Check sheet for the modelled part. Datum: model origin and axes. Units: mm. Face numbers are marked on the shaded views. A direction names the side the tool comes from. Give positions to 0.01 mm unless a question says otherwise; leave off trailing zeros. Order: outer loops, then holes, each group sorted by start corner. A loop starts at its lowest first (then second) coordinate and runs counter-clockwise, first axis right, second up. Notation, with made-up numbers: (19, 49) - (36, 49) arc R24 ccw to (36, 71) - close; hole circle Ø2 at (63.5, 32). An arc over 180 degrees is marked (long way). Answer in a Markdown table with one row per item.
from build123d import *

# Parameters (mm, degrees)
F1_DEPTH = 41.275
F0_W     = 25.4
F0_H     = 19.05
F2_DEPTH = 22.225
F4_DEPTH = 12.7
F5_R     = 6.35


with BuildPart() as f1:
    # F0 (on Front) → F1 (new body, symmetric)
    with BuildSketch(Plane.XZ):
        Polygon((-41.275, 9.525), (-41.275, -9.525), (41.275, -9.525), (41.275, 9.525), (22.225, 9.525), align=None)
    extrude(amount=F1_DEPTH, both=True)

    # F0 (on Front) → F2 (join, symmetric)
    with BuildSketch(Plane.XZ):
        with BuildLine():
            Line((22.225, 9.525), (41.275, 9.525))
            Line((41.275, 9.525), (41.275, 27.0002))
            ThreePointArc((41.275, 27.0002), (45.9246798487, 38.2255201513), (57.15, 42.8752))
            Line((57.15, 42.8752), (60.325, 42.8752))
            Line((60.325, 42.8752), (60.325, 61.9252))
            Line((60.325, 61.9252), (57.15, 61.9252))
            add(Edge.make_bspline(
                [(51.8284612448, 61.5173964429), (53.6256679067, 61.6821411581), (55.4011666766, 61.8176662229), (57.15, 61.9252)],
                knots=[106.0610091798, 106.0610091798, 106.0610091798, 106.0610091798, 111.5045361635, 111.5045361635, 111.5045361635, 111.5045361635], degree=3))
            ThreePointArc((51.8284612448, 61.5173964429), (30.6395269184, 49.7367441963), (22.225, 27.0002))
            Line((22.225, 27.0002), (22.225, 9.525))
        make_face()
        with Locations((73.025, 52.4002)):
            Rectangle(F0_W, F0_H)
    extrude(amount=F2_DEPTH, both=True)

    # F0 (on Front) → F3 (revolve)
    with BuildSketch(Plane.XZ):
        Polygon((85.725, 66.675), (85.725, 61.9252), (85.725, 42.8752), (85.725, 38.1), (111.125, 38.1), (111.125, 66.675), align=None)
    revolve(axis=Axis((85.725, 0, 54.7751), (0, 0, 1)))

    # F0 (on Front) → F4 (join)
    with BuildSketch(Plane.XZ):
        with BuildLine():
            add(Edge.make_bspline(
                [(-41.275, 9.525), (-26.4454266559, 44.0052587765), (16.8119080386, 58.3075307065), (51.8284612448, 61.5173964429)],
                knots=[0, 0, 0, 0, 106.0610091798, 106.0610091798, 106.0610091798, 106.0610091798], degree=3))
            Line((-41.275, 9.525), (22.225, 9.525))
            Line((22.225, 9.525), (22.225, 27.0002))
            ThreePointArc((22.225, 27.0002), (30.6395269184, 49.7367441963), (51.8284612448, 61.5173964429))
        make_face()
    extrude(amount=F4_DEPTH)

    # F5
    f5_edges = [f1.edges().sort_by_distance(p)[0] for p in [
        (41.275, -41.275, 0),
        (-41.275, -41.275, 0),
        (41.275, 41.275, 0),
        (-41.275, 41.275, 0),
    ]]
    fillet(f5_edges, radius=F5_R)


solid = f1.part
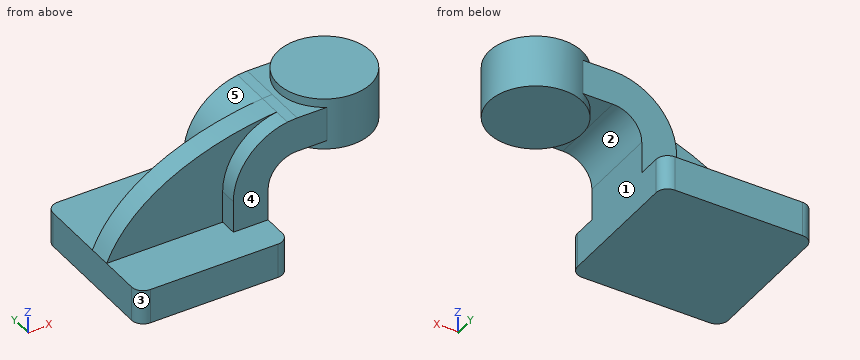
(1) Cross-section at B-B, the plane y = 33. Record the cut outline in (x, z) (3 decimals).
Geometry says:
| item | result |
|---|---|
| outline | (-41.275, -9.525) - (41.275, -9.525) - (41.275, 9.525) - (-41.275, 9.525) - close |
(2) Access from +Z, -Z, +X, -X, +Y, -Y to the whole of each face (thin tool, end or side, straight path). Record for the marked faces 1, 2, 3, 4 and 5.
Geometry says:
| item | result |
|---|---|
| face 1 | -Z, +X, +Y, -Y |
| face 2 | -Z, +Y, -Y |
| face 3 | +Z, -Z, -X, -Y |
| face 4 | +Z, -X, -Y |
| face 5 | +Z, -X, +Y |
(3) Thickness scan on L1, parallel to Z at x = -18, y = 24 (3 decimals); L2, parallel to Z at x = 57, y = 20.5; L3, parallel to X at y = -15, z = 8 (3 decimals). Record the ranges inside material, lowest first.
Geometry says:
| item | result |
|---|---|
| L1 | -9.525 to 9.525 |
| L2 | 42.87 to 61.92 |
| L3 | -41.275 to 41.275 |
(4) Gauge pin test, flat ends, axial feed: P1, Ø10.5, axis at y = -19.5, z = 19, coming from the -X side (3 decimals); P2, Ø2, axis at x = -13.5, z = 33, coming from the +Y side; P3, Ø6, axis at x = 78.5, y = -13.5, coming from the -Z side. Record the tip position at first contact, or that the pin passes through.
Geometry says:
| item | result |
|---|---|
| P1 | x = 22.225 |
| P2 | y = 0 |
| P3 | z = 38.1 |
(5) Cross-section at C-C, the plane x = 97. Record the cut outline in (y, z) (3 decimals).
Geometry says:
| item | result |
|---|---|
| outline | (-22.76, 38.1) - (22.76, 38.1) - (22.76, 66.675) - (-22.76, 66.675) - close |
(6) Cross-section at A-A, the plane z = 1.5. Record the cut outline in (x, y) (3 decimals), then the cut area to 3 significant figures.
Geometry says:
| item | result |
|---|---|
| outline | (-41.275, -34.925) arc R6.35 ccw to (-34.925, -41.275) - (34.925, -41.275) arc R6.35 ccw to (41.275, -34.925) - (41.275, 34.925) arc R6.35 ccw to (34.925, 41.275) - (-34.925, 41.275) arc R6.35 ccw to (-41.275, 34.925) - close |
| area | 6,780 mm² |
